Work out the finished part from the listing and answer in its coordinate system (mm). A direction names the side the tool comes from. Give positions to 0.01 mm unless a question says otherwise; leave off trailing zeros. Loops run counter-clockwise (first coordinate to the right, second up) from the corner with the lowest first, then second, coordinate; pieces in that order, holes last. Notation, with made-up numbers: (-29, -16) - (28, -16) arc R11 cw to (28, 0) - close; hole circle Ø8 at (-38.75, -3). An arc over 180 degrees is marked (long way). Use CSV: the item, a comma, the result in double quotes.
from build123d import *

# Parameters (mm, degrees)
SKETCH_R        = 30
PAD_DEPTH       = 2
SKETCH001_R     = 1.5
SKETCH001_R_2   = 0.5
PAD001_DEPTH    = 3
SKETCH009_R     = 4
PAD004_DEPTH    = 10
SKETCH010_R     = 2.25
POCKET004_DEPTH = 5.5
SKETCH011_R     = 4.25
POCKET005_DEPTH = 0.6
SKETCH012_W     = 20
SKETCH012_H     = 4
SKETCH012_W_2   = 2
SKETCH012_H_2   = 8
SKETCH012_W_3   = 8
SKETCH012_H_3   = 2
PAD005_DEPTH    = 5
SKETCH013_W     = 6
SKETCH013_H     = 4
SKETCH013_W_2   = 1
SKETCH013_H_2   = 0.75
POCKET006_DEPTH = 38.001
SKETCH014_W     = 6
SKETCH014_H     = 4
SKETCH014_W_2   = 1
SKETCH014_H_2   = 0.8
POCKET007_DEPTH = 2
CHAMFER_SIZE    = 0.5
SKETCH015_W     = 18
SKETCH015_H     = 4
SKETCH015_W_2   = 2
SKETCH015_H_2   = 0.8
POCKET008_DEPTH = 4
CHAMFER001_SIZE = 0.5
CHAMFER002_SIZE = 0.7
CHAMFER003_SIZE = 0.5
CHAMFER004_SIZE = 0.5
CHAMFER005_SIZE = 0.7


with BuildPart() as part:
    # Sketch (on DatumPlane) → Pad (new body)
    with BuildSketch(Plane(origin=(0, 0, -16.6), x_dir=(1, 0, 0), z_dir=(0, 0, -1))):
        Circle(SKETCH_R)
    extrude(amount=PAD_DEPTH)

    # Sketch001 (on Face2 of Pad) → Pad001 (join)
    with BuildSketch(Plane.XY.offset(-16.6)):
        with Locations((-16.1, 5.5)):
            Circle(SKETCH001_R)
        with Locations((-16.1, 5.5)):
            Circle(SKETCH001_R_2, mode=Mode.SUBTRACT)
        with Locations((-22.8, -6.4)):
            Circle(SKETCH001_R)
        with Locations((-22.8, -6.4)):
            Circle(SKETCH001_R_2, mode=Mode.SUBTRACT)
        with Locations((-15.5, -8.1)):
            Circle(SKETCH001_R)
        with Locations((-15.5, -8.1)):
            Circle(SKETCH001_R_2, mode=Mode.SUBTRACT)
        with Locations((-14.2, -12.7)):
            Circle(SKETCH001_R)
        with Locations((-14.2, -12.7)):
            Circle(SKETCH001_R_2, mode=Mode.SUBTRACT)
        with Locations((-14.6, -18.4)):
            Circle(SKETCH001_R)
        with Locations((-14.6, -18.4)):
            Circle(SKETCH001_R_2, mode=Mode.SUBTRACT)
        with Locations((-8.4, -22)):
            Circle(SKETCH001_R)
        with Locations((-8.4, -22)):
            Circle(SKETCH001_R_2, mode=Mode.SUBTRACT)
        with Locations((-5.2, -22.7)):
            Circle(SKETCH001_R)
        with Locations((-5.2, -22.7)):
            Circle(SKETCH001_R_2, mode=Mode.SUBTRACT)
        with Locations((10.240525, -14.05962)):
            Circle(SKETCH001_R)
        with Locations((10.240525, -14.05962)):
            Circle(SKETCH001_R_2, mode=Mode.SUBTRACT)
        with Locations((16.4, 5.2)):
            Circle(SKETCH001_R)
        with Locations((16.4, 5.2)):
            Circle(SKETCH001_R_2, mode=Mode.SUBTRACT)
        with Locations((23.6, 2.2)):
            Circle(SKETCH001_R)
        with Locations((23.6, 2.2)):
            Circle(SKETCH001_R_2, mode=Mode.SUBTRACT)
        with BuildLine():
            ThreePointArc((3.523134, -17.601478), (1.601478, -19.676866), (3.676866, -21.598522))
            Line((3.676866, -21.598522), (6.276866, -21.498522))
            ThreePointArc((6.276866, -21.498522), (8.198522, -19.423134), (6.123134, -17.501478))
            Line((3.523134, -17.601478), (6.123134, -17.501478))
        make_face()
        with Locations((3.6, -19.6)):
            Circle(SKETCH001_R_2, mode=Mode.SUBTRACT)
        with Locations((6.2, -19.5)):
            Circle(SKETCH001_R_2, mode=Mode.SUBTRACT)
    extrude(amount=PAD001_DEPTH)

    # Sketch009 (on Face2 of Pad001) → Pad004 (join)
    with BuildSketch(Plane.XY.offset(-16.6)):
        with Locations((22.083648, 12.75)):
            Circle(SKETCH009_R)
        with Locations((-22.083648, 12.75)):
            Circle(SKETCH009_R)
        with Locations((0, -25.5)):
            Circle(SKETCH009_R)
    extrude(amount=PAD004_DEPTH)

    # Sketch010 (on Face34 of Pad004) → Pocket004 (cut)
    with BuildSketch(Plane.XY.offset(-6.6)):
        with Locations((-22.083648, 12.75)):
            Circle(SKETCH010_R)
        with Locations((22.083648, 12.75)):
            Circle(SKETCH010_R)
        with Locations((0, -25.5)):
            Circle(SKETCH010_R)
    extrude(amount=-POCKET004_DEPTH, mode=Mode.SUBTRACT)

    # Sketch011 (on Face3 of Pocket004) → Pocket005 (cut)
    with BuildSketch(Plane(origin=(0, 0, -18.6), x_dir=(1, 0, 0), z_dir=(0, 0, -1))):
        with Locations((0, 21.75)):
            Circle(SKETCH011_R)
        with Locations((18.836053, -10.875)):
            Circle(SKETCH011_R)
        with Locations((-18.836053, -10.875)):
            Circle(SKETCH011_R)
    extrude(amount=-POCKET005_DEPTH, mode=Mode.SUBTRACT)

    # Sketch012 (on Face2 of Pocket005) → Pad005 (join)
    with BuildSketch(Plane.XY.offset(-16.6)):
        with Locations((0, 25)):
            Rectangle(SKETCH012_W, SKETCH012_H)
        with Locations((-7, 0)):
            Rectangle(SKETCH012_W_2, SKETCH012_H_2)
        with Locations((7, 0)):
            Rectangle(SKETCH012_W_2, SKETCH012_H_2)
        with Locations((0, -7)):
            Rectangle(SKETCH012_W_3, SKETCH012_H_3)
    extrude(amount=PAD005_DEPTH)

    # Sketch013 (on Face32 of Pad005) → Pocket006 (cut, through all)
    with BuildSketch(Plane(origin=(8, 0, -16.6), x_dir=(0, -1, 0), z_dir=(1, 0, 0))):
        with Locations((0, -2)):
            Rectangle(SKETCH013_W, SKETCH013_H)
        with Locations((0, -4.625)):
            Rectangle(SKETCH013_W_2, SKETCH013_H_2)
    extrude(amount=-POCKET006_DEPTH, mode=Mode.SUBTRACT)

    # Sketch014 (on Face29 of Pocket006) → Pocket007 (cut)
    with BuildSketch(Plane(origin=(0, -8, -16.6), x_dir=(-1, 0, 0), z_dir=(0, -1, 0))):
        with Locations((0, -2)):
            Rectangle(SKETCH014_W, SKETCH014_H)
        with Locations((0, -4.6)):
            Rectangle(SKETCH014_W_2, SKETCH014_H_2)
    extrude(amount=-POCKET007_DEPTH, mode=Mode.SUBTRACT)

    # Chamfer
    chamfer_edges = [part.edges().sort_by_distance(p)[0] for p in [
        (-7, 0.5, -11.6),
        (-7, -0.5, -11.6),
        (-0.5, -7, -11.6),
        (0.5, -7, -11.6),
        (7, -0.5, -11.6),
        (7, 0.5, -11.6),
    ]]
    chamfer(chamfer_edges, length=CHAMFER_SIZE)

    # Sketch015 (on Face17 of Chamfer) → Pocket008 (cut)
    with BuildSketch(Plane(origin=(0, 23, -16.6), x_dir=(-1, 0, 0), z_dir=(0, -1, 0))):
        with Locations((0, -2)):
            Rectangle(SKETCH015_W, SKETCH015_H)
        with Locations((0, -4.6)):
            Rectangle(SKETCH015_W_2, SKETCH015_H_2)
    extrude(amount=-POCKET008_DEPTH, mode=Mode.SUBTRACT)

    # Chamfer001
    chamfer001_edges = [part.edges().sort_by_distance(p)[0] for p in [
        (-1, 25, -11.6),
        (1, 25, -11.6),
    ]]
    chamfer(chamfer001_edges, length=CHAMFER001_SIZE)

    # Chamfer002
    chamfer002_edges = [part.edges().sort_by_distance(p)[0] for p in [
        (10, 25, -11.6),
        (-10, 25, -11.6),
        (-7, 4, -11.6),
        (-7, -4, -11.6),
        (-4, -7, -11.6),
        (4, -7, -11.6),
        (7, -4, -11.6),
        (7, 4, -11.6),
    ]]
    chamfer(chamfer002_edges, length=CHAMFER002_SIZE)

    # Chamfer003
    chamfer003_edges = [part.edges().sort_by_distance(p)[0] for p in [
        (-24.333648, 12.75, -6.6),
        (19.833648, 12.75, -6.6),
        (-2.25, -25.5, -6.6),
    ]]
    chamfer(chamfer003_edges, length=CHAMFER003_SIZE)

    # Chamfer004
    chamfer004_edges = [part.edges().sort_by_distance(p)[0] for p in [
        (-16.6, 5.5, -13.6),
        (15.9, 5.2, -13.6),
        (23.1, 2.2, -13.6),
        (9.740525, -14.05962, -13.6),
        (5.7, -19.5, -13.6),
        (3.1, -19.6, -13.6),
        (-8.9, -22, -13.6),
        (-5.7, -22.7, -13.6),
        (-15.1, -18.4, -13.6),
        (-14.7, -12.7, -13.6),
        (-16, -8.1, -13.6),
        (-23.3, -6.4, -13.6),
    ]]
    chamfer(chamfer004_edges, length=CHAMFER004_SIZE)

    # Chamfer005
    chamfer005_edges = [part.edges().sort_by_distance(p)[0] for p in [
        (-24.3, -6.4, -16.6),
        (-17.6, 5.5, -16.6),
        (-17, -8.1, -16.6),
        (-15.7, -12.7, -16.6),
        (-16.1, -18.4, -16.6),
        (8.740525, -14.05962, -16.6),
        (14.9, 5.2, -16.6),
        (22.1, 2.2, -16.6),
        (8.198522, -19.423134, -16.6),
        (4, -7, -16.6),
        (7, -4, -16.6),
        (-7, -4, -16.6),
        (3.5, -8, -16.6),
        (-3.5, -8, -16.6),
        (-3, -7, -16.6),
        (7, 3, -16.6),
        (8, 3.5, -16.6),
        (8, -3.5, -16.6),
        (-6, -3.5, -16.6),
        (-6, 3.5, -16.6),
        (-7, 3, -16.6),
        (6, 3.5, -16.6),
        (-8, -3.5, -16.6),
        (-8, 3.5, -16.6),
        (-4, -7, -16.6),
        (3, -7, -16.6),
        (6, -3.5, -16.6),
        (7, -3, -16.6),
        (7, 4, -16.6),
        (-7, 4, -16.6),
        (-7, -3, -16.6),
        (-3.5, -6, -16.6),
        (3.5, -6, -16.6),
        (-9.5, 23, -16.6),
        (-10, 25, -16.6),
        (-9.5, 27, -16.6),
        (-9, 25, -16.6),
        (10, 25, -16.6),
        (9.5, 27, -16.6),
        (9, 25, -16.6),
        (9.5, 23, -16.6),
    ]]
    chamfer(chamfer005_edges, length=CHAMFER005_SIZE)


solid = part.part
Item 1: Find the intervals of material crossed by line 1 (Y direction, x = 0, z = -18.3); line 2 (Y direction, x = 16.4, z = -15.45); line 3 (Y direction, x = 23.6, z = -15.85), in increasing order.
Determined:
line 1,"y = -30 to -26, -17.5 to 30"
line 2,"y = 3.7 to 4.7, 5.7 to 6.7"
line 3,"y = 0.7 to 1.7, 2.7 to 3.7, 9.05 to 16.45"
Item 2: A cutting plane is placed at A-A on z = -9.5. Determine the outline of the cut face in (x, y).
Determined:
outline,"circle Ø8 at (-22.08, 12.75); circle Ø8 at (0, -25.5); circle Ø8 at (22.08, 12.75); hole circle Ø4.5 at (-22.08, 12.75); hole circle Ø4.5 at (0, -25.5); hole circle Ø4.5 at (22.08, 12.75)"
Item 3: For faces 1 (the flat face through (0, 25, -12.6)), 2 (the flat face through (10, 25, -14)), 3 (the flat face through (1, -6, -12)), 4 (the flat face through (-7, 0, -12.6)), determine the directions among +Z, -Z, +X, -X, +Y, -Y from which every point of the face is accessible in a straight line to the end or side of a thin tool.
Determined:
face 1,"+Y"
face 2,"+Z, +X, +Y"
face 3,"+Z, +X"
face 4,"+X, -X"
Item 4: The mould has two halves that part along Z. Classify faces 5 (the flat face through (-4, -7, -14)), 6 (the flat face through (5, -20, -13.6)), 7 (the flat face through (7, 0, -12.6)): pulls with the +Z half, pulls with the -Z half, needs draft (parallel to the pull), parting line crosses it, or undercut.
Determined:
face 5,"needs draft"
face 6,"pulls with the +Z half"
face 7,"undercut"
Item 5: Given P1, Ø0.9, axis at x = -16.5, y = 5.5, coming from the +Z side; P2, Ø2, axis at x = -0.5, z = -14, coming from the -Y side; P3, Ø2, axis at y = -18.5, z = -11.5, coming from the -X side; P4, Ø2, axis at x = -0.5, z = -14, coming from the +Y side, each flat-ended and moving along its own axis, determine where each tip first touches the part or whether it passes through.
Determined:
P1,"stops at z = -13.75"
P2,"stops at y = -29.5"
P3,"passes through"
P4,"stops at y = -21.5"
